Could you check a few things on this model? Use its own coordinates, in mm. A direction names the side the tool comes from. Coordinates: 2 decimals unless noted, no trailing zeros. Order: outer loops, then holes, each group sorted by start corner. A loop starts at its lowest first (then second) coordinate and runs counter-clockwise, first axis right, second up. Notation, with made-up numbers: (75.5, 58.5) -> (90.5, 58.5) arc R28 ccw to (90.5, 89.5) -> close; hole circle Ø2 at (-5.5, 66). An arc over 180 degrees is marked (long way). Return JSON: item names as keys, results as strings. Group by question number.
from build123d import *

# Parameters (mm, degrees)
BOSS_EXTRUDE1_DEPTH   = 27
FILLET1_R             = 3
FILLET2_R             = 3
SKETCH3_R             = 1.75
BOSS_EXTRUDE2_DEPTH   = 7
SKETCH4_R             = 0.5
BOSS_EXTRUDE3_DEPTH   = 7
BOSS_EXTRUDE3_2_DEPTH = 7
BOSS_EXTRUDE3_3_DEPTH = 7
BOSS_EXTRUDE3_4_DEPTH = 7


with BuildPart() as part:
    # Sketch1 → Boss-Extrude1 (new body)
    with BuildSketch(Plane.XY):
        with BuildLine():
            Line((-10, -11), (-10, 11))
            ThreePointArc((-10, 11), (0, 15), (10, 11))
            Line((10, 11), (10, -11))
            ThreePointArc((10, -11), (0, -15), (-10, -11))
        make_face()
    extrude(amount=BOSS_EXTRUDE1_DEPTH)

    # Fillet1
    fillet1_edges = [part.edges().sort_by_distance(p)[0] for p in [
        (10, 11, 13.5),
        (10, -11, 13.5),
        (-10, -11, 13.5),
        (-10, 11, 13.5),
    ]]
    fillet(fillet1_edges, radius=FILLET1_R)

    # Fillet2
    fillet2_edges = [part.edges().sort_by_distance(p)[0] for p in [
        (10, 0, 27),
        (0, -15, 27),
        (0, 15, 27),
        (-10, 0, 27),
        (9.690563219, 10.951121401, 27),
        (-9.690563219, 10.951121401, 27),
        (-9.690563219, -10.951121401, 27),
        (9.690563219, -10.951121401, 27),
    ]]
    fillet(fillet2_edges, radius=FILLET2_R)

    # Sketch3 → Boss-Extrude2 (add)
    with BuildSketch(Plane(origin=(0, 0, 0), x_dir=(-1, 0, 0), z_dir=(0, 0, -1))):
        Circle(SKETCH3_R)
    extrude(amount=BOSS_EXTRUDE2_DEPTH)


with BuildPart() as body_2:
    # Sketch4 → Boss-Extrude3 (new body)
    with BuildSketch(Plane(origin=(0, 0, 0), x_dir=(-1, 0, 0), z_dir=(0, 0, -1))):
        with Locations((-5.75, 0)):
            Circle(SKETCH4_R)
    extrude(amount=BOSS_EXTRUDE3_DEPTH)


with BuildPart() as body_3:
    # Sketch4 → Boss-Extrude3 2 (new body)
    with BuildSketch(Plane(origin=(0, 0, 0), x_dir=(-1, 0, 0), z_dir=(0, 0, -1))):
        with Locations((-5.75, 4.5)):
            Circle(SKETCH4_R)
    extrude(amount=BOSS_EXTRUDE3_2_DEPTH)


with BuildPart() as body_4:
    # Sketch4 → Boss-Extrude3 3 (new body)
    with BuildSketch(Plane(origin=(0, 0, 0), x_dir=(-1, 0, 0), z_dir=(0, 0, -1))):
        with Locations((-4, 8)):
            Circle(SKETCH4_R)
    extrude(amount=BOSS_EXTRUDE3_3_DEPTH)


with BuildPart() as body_5:
    # Sketch4 → Boss-Extrude3 4 (new body)
    with BuildSketch(Plane(origin=(0, 0, 0), x_dir=(-1, 0, 0), z_dir=(0, 0, -1))):
        with Locations((0, 9)):
            Circle(SKETCH4_R)
    extrude(amount=BOSS_EXTRUDE3_4_DEPTH)


with BuildPart() as body_6:
    # Mirror1: mirrored copy
    add(body_4.part.mirror(Plane(origin=(0, 0, 0), x_dir=(0, 0, 1), z_dir=(1, 0, 0))))


with BuildPart() as body_7:
    # Mirror1 2: mirrored copy
    add(body_3.part.mirror(Plane(origin=(0, 0, 0), x_dir=(0, 0, 1), z_dir=(1, 0, 0))))


with BuildPart() as body_8:
    # Mirror1 3: mirrored copy
    add(body_2.part.mirror(Plane(origin=(0, 0, 0), x_dir=(0, 0, 1), z_dir=(1, 0, 0))))


with BuildPart() as body_9:
    # Mirror2: mirrored copy
    add(body_3.part.mirror(Plane.ZX))


with BuildPart() as body_10:
    # Mirror2 2: mirrored copy
    add(body_4.part.mirror(Plane.ZX))


with BuildPart() as body_11:
    # Mirror2 3: mirrored copy
    add(body_5.part.mirror(Plane.ZX))


with BuildPart() as body_12:
    # Mirror2 4: mirrored copy
    add(body_6.part.mirror(Plane.ZX))


with BuildPart() as body_13:
    # Mirror2 5: mirrored copy
    add(body_7.part.mirror(Plane.ZX))


with BuildPart() as body_2_1:
    add(body_2.part)

    # Combine1: union body 5, body 7, body 9, body 13, body 3, body 6, body 12, body 4, body 11, body 8, body 10, part
    add(body_5.part)
    add(body_7.part)
    add(body_9.part)
    add(body_13.part)
    add(body_3.part)
    add(body_6.part)
    add(body_12.part)
    add(body_4.part)
    add(body_11.part)
    add(body_8.part)
    add(body_10.part)
    add(part.part)


solid = body_2_1.part
Q1. I want a section at C-C on x = 0. Please give me the cut outline in (y, z).
Q2. I'm going to push flat-ended pins straight in: pin 1 Ø3 at (x, z) = (-7, 12) entering from +Y; pin 2 Ø12 at (y, z) = (-10.5, 11.5) entering from -X; pin 3 Ø1 at (x, z) = (-2, 18) entering from +Y; pin 4 Ø5 at (x, z) = (7.5, 9) entering from -Y. Where does each tip first touch, or does it pass through?
Q3. I want a section at A-A on y = 0. Please give me the cut outline in (x, z), and give its area (3 significant figures).
Q4. I want a section at B-B on z = 4.5. Please give me the cut outline in (x, y).
Q5. I need wall thicknesses on line 1 along Z through (x, y) = (-4.5, -4.5); line 2 along X through (y, z) = (-9, -3.5); line 3 along Y through (x, z) = (3.75, -1.5). Which ranges of each line are inside material? Lowest first, please. Write a range as from..to.
Q6. On a 3-axis mill with a long thin cutter (end or side, diameter ignored), from which of +Z, -Z, +X, -X, +Y, -Y can I reach the whole of each face in a straight line? I mean faces 4 (the flat face through (4, -8, -7)), 5 (the cylindrical face through (-1.617, -0.67, -3.451)). Say none if no direction works.
Q7. We'd pull the mould along X, two halves only. Please class faces 1 (the cylindrical face through (4.108, -7.512, -3.451)), 2 (the flat face through (4, 8, -7)), 3 (the flat face through (-10, 0, 12)): pulls with the +X half, pulls with the -X half, needs draft (parallel to the pull), parting line crosses it, or undercut.
Q8. I want a section at D-D on y = 8. Please give me the cut outline in (x, z).
Response values:
{
 "1": {"outline": "(-15, 0) -> (-9.5, 0) -> (-9.5, -7) -> (-8.5, -7) -> (-8.5, 0) -> (-1.75, 0) -> (-1.75, -7) -> (1.75, -7) -> (1.75, 0) -> (8.5, 0) -> (8.5, -7) -> (9.5, -7) -> (9.5, 0) -> (15, 0) -> (15, 24) arc R3 ccw to (12, 27) -> (-12, 27) arc R3 ccw to (-15, 24) -> close"},
 "2": {"pin 1": "stops at y = 13.92", "pin 2": "stops at x = -10", "pin 3": "stops at y = 14.92", "pin 4": "stops at y = -14.11"},
 "3": {"outline": "(-10, 0) -> (-6.25, 0) -> (-6.25, -7) -> (-5.25, -7) -> (-5.25, 0) -> (-1.75, 0) -> (-1.75, -7) -> (1.75, -7) -> (1.75, 0) -> (5.25, 0) -> (5.25, -7) -> (6.25, -7) -> (6.25, 0) -> (10, 0) -> (10, 24) arc R3 ccw to (7, 27) -> (-7, 27) arc R3 ccw to (-10, 24) -> close", "area": "575 mm²"},
 "4": {"outline": "(-10, -9.62) arc R3 ccw to (-8.83, -12) arc R14.5 ccw to (8.83, -12) arc R3 ccw to (10, -9.62) -> (10, 9.62) arc R3 ccw to (8.83, 12) arc R14.5 ccw to (-8.83, 12) arc R3 ccw to (-10, 9.62) -> close"},
 "5": {"line 1": "z = 0..27", "line 2": "x = -0.5..0.5", "line 3": "y = -8.43..-7.57, 7.57..8.43"},
 "6": {"face 4": "-Z, +X, -X, +Y, -Y", "face 5": "-Z"},
 "7": {"face 1": "undercut", "face 2": "needs draft", "face 3": "pulls with the -X half"},
 "8": {"outline": "(-10, 0) -> (-4.5, 0) -> (-4.5, -7) -> (-3.5, -7) -> (-3.5, 0) -> (3.5, 0) -> (3.5, -7) -> (4.5, -7) -> (4.5, 0) -> (10, 0) -> (10, 24) arc R3 ccw to (7, 27) -> (-7, 27) arc R3 ccw to (-10, 24) -> close"}
}
